Geometry: final body of the model. Coordinates: model frame, mm. Coordinates: 2 decimals unless noted, no trailing zeros. Loops run counter-clockwise (first coordinate to the right, second up) from the corner with the lowest first, then second, coordinate; pieces in that order, holes last. Notation, with made-up numbers: (7.5, 2) -> (55.5, 2) arc R19 ccw to (55.5, 8) -> close; hole circle Ø8 at (45.25, 50.25). An arc over 180 degrees is marked (long way). One line per item, written item: value. Start each with the question number.
Autodesk Fusion 360 part; units mm, degrees
sketch "Sketch1" plane through (0, 0, 0) normal (0, 0, 1) x (1, 0, 0)
  line L0 (-0.9, 44.4476) -> (72, 44.4476)
  line L1 (72, 44.4476) -> (72, 2.6476)
  line L2 (72, 2.6476) -> (-0.9, 2.6476)
  line L3 (-0.9, 2.6476) -> (-0.9, 44.4476)
  line L4 (-0.9, 23.5476) -> (72, 23.5476) construction
  line L5 (-0.9, 28.5476) -> (-4.6, 28.5476)
  line L6 (-5.9, 27.2476) -> (-5.9, 19.8476)
  line L7 (-4.6, 18.5476) -> (-0.9, 18.5476)
  line L8 (-0.9, 18.5476) -> (-0.9, 28.5476)
  arc A0 (-4.6, 28.5476) -> (-5.9, 27.2476) centre (-4.6, 27.2476) ccw
  arc A1 (-5.9, 19.8476) -> (-4.6, 18.5476) centre (-4.6, 19.8476) ccw
  line L9 (72, 36.7476) -> (66.7, 36.7476)
  line L10 (66.7, 36.7476) -> (66.7, 31.7476)
  line L11 (66.7, 31.7476) -> (72, 31.7476)
  line L12 (72, 31.7476) -> (72, 36.7476)
  line L13 (46, 16.0476) -> (48.5, 16.0476)
  line L14 (48.5, 16.0476) -> (48.5, 11.0476)
  line L15 (48.5, 11.0476) -> (46, 11.0476)
  line L16 (46, 11.0476) -> (46, 16.0476)
  line L17 (9.1, 12.0476) -> (13.7, 12.0476)
  line L18 (13.7, 12.0476) -> (13.7, 9.7476)
  line L19 (13.7, 9.7476) -> (9.1, 9.7476)
  line L20 (9.1, 9.7476) -> (9.1, 12.0476)
  point P0 (-5.9, 28.5476)
  point P1 (-5.9, 18.5476)
  dimension "d1" = 72.9
  dimension "d2" = 41.8
  dimension "d7" = 10
  dimension "d8" = 5
  dimension "d9" = 1.3
  dimension "d10" = 5.3
  dimension "d11" = 5
  dimension "d12" = 7.7
  dimension "d13" = 2.5
  dimension "d14" = 5
  dimension "d15" = 8.4
  dimension "d16" = 23.5
  dimension "d17" = 2.3
  dimension "d18" = 7.1
  dimension "d19" = 10
  dimension "d20" = 14.6
extrude "Extrude1" add sketch "Sketch1" along normal blind 1 contours L0 L1 L2 L3 L8 L9 L10 L11 | L3 L5 L6 L7 L8 A0 A1
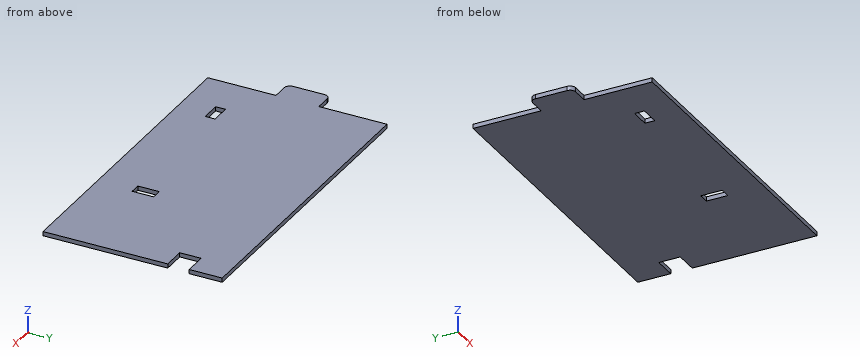
1. Section C-C on y = 39. Return the cut outline in (x, z), plus the area to 3 significant figures.
2. Pin query (flat end, axial travel): pin 1 Ø10 at (x, y) = (15, 21.5) entering from -Z; pin 2 Ø0.5 at (y, z) = (11, 0.5) entering from -X; pin 3 Ø0.5 at (x, z) = (-2, 0.5) entering from -Y. Return the tip coordinate at first contact, or that it passes through.
3. Section B-B on y = 34. Return the cut outline in (x, z).
4. Section A-A on z = 0.7. Return the cut outline in (x, y).
5. Line query: L1, parallel to Y at x = 10.5, z = 0.6; L2, parallel to Y at x = 46.5, z = 0.85; L3, parallel to X at y = 14, z = 0.3. Output: solid intervals per line, ascending. Write a range as [from, to].
Checks:
1. outline: (-0.9, 0) -> (72, 0) -> (72, 1) -> (-0.9, 1) -> close
1. area: 72.9 mm²
2. pin 1: z = 0
2. pin 2: x = -0.9
2. pin 3: y = 18.55
3. outline: (-0.9, 0) -> (66.7, 0) -> (66.7, 1) -> (-0.9, 1) -> close
4. outline: (-5.9, 19.85) arc R1.3 ccw to (-4.6, 18.55) -> (-0.9, 18.55) -> (-0.9, 2.65) -> (72, 2.65) -> (72, 31.75) -> (66.7, 31.75) -> (66.7, 36.75) -> (72, 36.75) -> (72, 44.45) -> (-0.9, 44.45) -> (-0.9, 28.55) -> (-4.6, 28.55) arc R1.3 ccw to (-5.9, 27.25) -> close; hole (9.1, 9.75) -> (13.7, 9.75) -> (13.7, 12.05) -> (9.1, 12.05) -> close; hole (46, 11.05) -> (48.5, 11.05) -> (48.5, 16.05) -> (46, 16.05) -> close
5. L1: [2.65, 9.75], [12.05, 44.45]
5. L2: [2.65, 11.05], [16.05, 44.45]
5. L3: [-0.9, 46], [48.5, 72]
